```python
from build123d import *
from build123d.topology import SkipClean

# Parameters (mm, degrees)
SKETCH1_R           = 15
SKETCH1_R_2         = 10
SKETCH1_R_3         = 6
BOSS_EXTRUDE1_DEPTH = 5
BOSS_EXTRUDE2_START = 2.5
SKETCH2_R           = 15
SKETCH2_R_2         = 10
BOSS_EXTRUDE2_DEPTH = 2.5
BOSS_EXTRUDE4_START = 3
BOSS_EXTRUDE4_DEPTH = 3
SKETCH4_R           = 7
SKETCH4_R_2         = 6
BOSS_EXTRUDE5_DEPTH = 1.75


with BuildPart() as part:
    # Sketch1 → Boss-Extrude1 (new body)
    # profile 1 of 2: a face of its own
    with BuildSketch(Plane.XY):
        Circle(SKETCH1_R)
        Circle(SKETCH1_R_2, mode=Mode.SUBTRACT)
    # profile 2 of 2: a face of its own
    with BuildSketch(Plane.XY):
        Circle(SKETCH1_R_2)
        Circle(SKETCH1_R_3, mode=Mode.SUBTRACT)
    extrude(amount=-BOSS_EXTRUDE1_DEPTH)

    # Sketch2 → Boss-Extrude2 (add)
    with BuildSketch(Plane.XY.offset(BOSS_EXTRUDE2_START)):
        Circle(SKETCH2_R)
        Circle(SKETCH2_R_2, mode=Mode.SUBTRACT)
    extrude(amount=-BOSS_EXTRUDE2_DEPTH)

    # Sketch3 → Boss-Extrude4 (add)
    with SkipClean():  # the faces are left unmerged after this step: merging them gives an invalid solid
        with BuildSketch(Plane.XY.offset(2.5).offset(BOSS_EXTRUDE4_START)):
            with BuildLine():
                ThreePointArc((-2.290603582, -14.824072829), (0, -15), (2.290603582, -14.824072829))
                ThreePointArc((2.290603582, -14.824072829), (3.086155614, -13.560105094), (3.235238064, -12.074072829))
                ThreePointArc((3.235238064, -12.074072829), (2.788392741, -10.80499404), (1.867509855, -9.824072829))
                ThreePointArc((1.867509855, -9.824072829), (0, -10), (-1.867509855, -9.824072829))
                ThreePointArc((-1.867509855, -9.824072829), (-2.788392741, -10.80499404), (-3.235238064, -12.074072829))
                ThreePointArc((-3.235238064, -12.074072829), (-3.086155614, -13.560105094), (-2.290603582, -14.824072829))
            make_face()
            with BuildLine():
                ThreePointArc((-14.806366496, -2.402396967), (-14.265847744, -4.635254916), (-13.390695627, -6.759383893))
                ThreePointArc((-13.390695627, -6.759383893), (-11.942751779, -7.125411327), (-10.483382099, -6.807987938))
                ThreePointArc((-10.483382099, -6.807987938), (-9.414499246, -5.990845869), (-8.766156198, -4.811912875))
                ThreePointArc((-8.766156198, -4.811912875), (-9.510565163, -3.090169944), (-9.920340763, -1.259698041))
                ThreePointArc((-9.920340763, -1.259698041), (-11.137820734, -0.687007696), (-12.482869184, -0.654199453))
                ThreePointArc((-12.482869184, -0.654199453), (-13.850100843, -1.255194512), (-14.806366496, -2.402396967))
            make_face()
            with BuildLine():
                ThreePointArc((-6.860234162, 13.339309849), (-8.816778784, 12.135254916), (-10.566508613, 10.64654384))
                ThreePointArc((-10.566508613, 10.64654384), (-10.467182133, 9.15635871), (-9.714324518, 7.866504888))
                ThreePointArc((-9.714324518, 7.866504888), (-8.606873263, 7.102447672), (-7.285292336, 6.850147121))
                ThreePointArc((-7.285292336, 6.850147121), (-5.877852523, 8.090169944), (-4.263597916, 9.045536624))
                ThreePointArc((-4.263597916, 9.045536624), (-4.095159033, 10.380399934), (-4.479599369, 11.669755331))
                ThreePointArc((-4.479599369, 11.669755331), (-5.473677455, 12.784352223), (-6.860234162, 13.339309849))
            make_face()
            with BuildLine():
                ThreePointArc((10.566508613, 10.64654384), (8.816778784, 12.135254916), (6.860234162, 13.339309849))
                ThreePointArc((6.860234162, 13.339309849), (5.473677455, 12.784352223), (4.479599369, 11.669755331))
                ThreePointArc((4.479599369, 11.669755331), (4.095159033, 10.380399934), (4.263597916, 9.045536624))
                ThreePointArc((4.263597916, 9.045536624), (5.877852523, 8.090169944), (7.285292336, 6.850147121))
                ThreePointArc((7.285292336, 6.850147121), (8.606873263, 7.102447672), (9.714324518, 7.866504888))
                ThreePointArc((9.714324518, 7.866504888), (10.467182133, 9.15635871), (10.566508613, 10.64654384))
            make_face()
            with BuildLine():
                ThreePointArc((13.390695627, -6.759383893), (14.265847744, -4.635254916), (14.806366496, -2.402396967))
                ThreePointArc((14.806366496, -2.402396967), (13.850100843, -1.255194512), (12.482869184, -0.654199453))
                ThreePointArc((12.482869184, -0.654199453), (11.137820734, -0.687007696), (9.920340763, -1.259698041))
                ThreePointArc((9.920340763, -1.259698041), (9.510565163, -3.090169944), (8.766156198, -4.811912875))
                ThreePointArc((8.766156198, -4.811912875), (9.414499246, -5.990845869), (10.483382099, -6.807987938))
                ThreePointArc((10.483382099, -6.807987938), (11.942751779, -7.125411327), (13.390695627, -6.759383893))
            make_face()
        extrude(amount=-BOSS_EXTRUDE4_DEPTH)

    # Sketch4 → Boss-Extrude5 (add)
    with SkipClean():  # the faces are left unmerged after this step: merging them gives an invalid solid
        with BuildSketch(Plane(origin=(0, 0, -5), x_dir=(-1, 0, 0), z_dir=(0, 0, -1))):
            with Locations(Location((0, 0, 0), (0, 0, 180))):
                Circle(SKETCH4_R)
            with Locations(Location((0, 0, 0), (0, 0, 180))):
                Circle(SKETCH4_R_2, mode=Mode.SUBTRACT)
        extrude(amount=BOSS_EXTRUDE5_DEPTH)


solid = part.part
```
The model under review builds one solid part; all positions refer to its coordinate system, in mm. A direction names the side the tool comes from. Round coordinates to 2 decimals unless told otherwise and drop trailing zeros. Write each loop counter-clockwise with the first axis right and the second up, starting at its lowest first coordinate (ties: lowest second). Pieces come first, ordered by that corner, then holes. Notation, with made-up numbers: (76, -9) - (81, -9) arc R7 ccw to (81, 2) - close; hole circle Ø10 at (83.5, 51.25). An arc over 180 degrees is marked (long way). Answer as CSV lines item,"result". Start each with the question number.
(1) We need section C-C on x = 0. State the section outline as (y, z) points.
(2) We need section A-A on y = 0. State the section outline as (x, z) points.
(3) For faces 4 (the flat face through (6.5, -3.1, -5)), 5 (the flat face through (0, -7, 0)), 6 (the flat face through (7, 10, 5.5)), list the 3-axis set-ups (+Z, -Z, +X, -X, +Y, -Y) from which the entire face can be reached by the end or side of a thin tool; tool diameter is ignored.
(4) We need section D-D on z = -4. State the section outline as (x, y) points.
(5) We need section B-B on z = 4.5. State the section outline as (x, y) points.
(6) Draft analysis for pull direction X (two halves, no side actions). For faces 1 (the flat face through (0, 13, 2.5)), 2 (the cylindrical face through (6.466, 2.681, -5.863)), 3 (the flat face through (12, -4, 5.5)), state which applies: pulls with the +X half, pulls with the -X half, needs draft (parallel to the pull), parting line crosses it, or undercut.
(7) To check wall thickness, follow line 1 (Y direction, x = 0, z = -6.1); line 2 (X direction, y = 0, z = 1.25). State the ranges of each line that lie inside material, in increasing order.
(8) For pin 1 Ø6 at (y, z) = (7.5, 1) entering from +X; pin 2 Ø11 at (x, y) = (0, 0) entering from +Z; pin 3 Ø4 at (x, y) = (12, 3) entering from +Z; pin 4 Ø1.5 at (y, z) = (4.5, 2) entering from -X, all flat-tipped, find the tip position at first contact; note any pin that passes through.
Worked answers:
1,outline,"(-15, -5) - (-7, -5) - (-7, -6.75) - (-6, -6.75) - (-6, 0) - (-10, 0) - (-10, 5.5) - (-15, 5.5) - close; (6, -6.75) - (7, -6.75) - (7, -5) - (15, -5) - (15, 2.5) - (10, 2.5) - (10, 0) - (6, 0) - close"
2,outline,"(-15, -5) - (-7, -5) - (-7, -6.75) - (-6, -6.75) - (-6, 0) - (-10, 0) - (-10, 2.5) - (-15, 2.5) - close; (6, -6.75) - (7, -6.75) - (7, -5) - (15, -5) - (15, 2.5) - (10, 2.5) - (10, 0) - (6, 0) - close"
3,face 4,"-Z"
3,face 5,"+Z"
3,face 6,"+Z, +X, -X, +Y, -Y"
4,outline,"circle Ø30 at (0, 0); hole circle Ø12 at (0, 0)"
5,outline,"(-14.81, -2.4) arc R15 ccw to (-13.39, -6.76) arc R3.26 ccw to (-8.77, -4.81) arc R10 cw to (-9.92, -1.26) arc R3.26 ccw to start; (-10.57, 10.65) arc R3.26 ccw to (-7.29, 6.85) arc R10 cw to (-4.26, 9.05) arc R3.26 ccw to (-6.86, 13.34) arc R15 ccw to start; (-2.29, -14.82) arc R15 ccw to (2.29, -14.82) arc R3.26 ccw to (1.87, -9.82) arc R10 cw to (-1.87, -9.82) arc R3.26 ccw to start; (4.26, 9.05) arc R10 cw to (7.29, 6.85) arc R3.26 ccw to (10.57, 10.65) arc R15 ccw to (6.86, 13.34) arc R3.26 ccw to start; (8.77, -4.81) arc R3.26 ccw to (13.39, -6.76) arc R15 ccw to (14.81, -2.4) arc R3.26 ccw to (9.92, -1.26) arc R10 cw to start"
6,face 1,"undercut"
6,face 2,"parting line crosses it"
6,face 3,"needs draft"
7,line 1,"-7 to -6, 6 to 7"
7,line 2,"-15 to -10, 10 to 15"
8,pin 1,"x = 14.31"
8,pin 2,"through"
8,pin 3,"z = 2.5"
8,pin 4,"x = -14.52"
